from build123d import *

# Parameters (mm, degrees)
FILLET1_R               = 0.1
FILLET2_R               = 0.15
HEX_2_DEPTH             = 1.3
CUT_EXTRUDE1_DEPTH      = 14.569266765
CUT_EXTRUDE1_DEPTH_BACK = 14.569266765
SKETCH4_R               = 0.5


with BuildPart() as part:
    # BodySke → Base-Revolve (revolve)
    with BuildSketch(Plane.XY, mode=Mode.PRIVATE) as base_revolve_sk:
        Polygon((0, 0), (0, 2.75), (3, 2.75), (3, 1.5), (12.7195, 1.5), (13, 1.2195), (13, 0), align=None)
    revolve(base_revolve_sk.sketch.rotate(Axis((-31.75, 0, 0), (1, 0, 0)), 90), axis=Axis((-31.75, 0, 0), (1, 0, 0)))

    # Fillet1
    fillet1_edges = [part.edges().sort_by_distance(p)[0] for p in [
        (3, 0, -1.5),
    ]]
    fillet(fillet1_edges, radius=FILLET1_R)

    # Fillet2
    fillet2_edges = [part.edges().sort_by_distance(p)[0] for p in [
        (0, 0, -2.75),
    ]]
    fillet(fillet2_edges, radius=FILLET2_R)

    # Sketch2 → Hex-PreBroach (revolve, cut)
    with BuildSketch(Plane.XY, mode=Mode.PRIVATE) as hex_prebroach_sk:
        Polygon((0, 1.28), (1.3, 1.28), (2.039008345, 0), (0, 0), align=None)
    revolve(hex_prebroach_sk.sketch.rotate(Axis((0, 0, 0), (1, 0, 0)), 90), axis=Axis((0, 0, 0), (1, 0, 0)), mode=Mode.SUBTRACT)

    # Sketch3 → Hex 2 (cut)
    with BuildSketch(Plane(origin=(0, 0, 0), x_dir=(0, 0.500000000000001, 0.866025403784438), z_dir=(-1, 0, 0))):
        Polygon((0.739008345, 1.28), (-0.739008345, 1.28), (-1.478016689, 0), (-0.739008345, -1.28), (0.739008345, -1.28), (1.478016689, 0), align=None)
    extrude(amount=-HEX_2_DEPTH, mode=Mode.SUBTRACT)

    # Sketch4 → Cut-Extrude1 (cut, two sides: drawn at the far end of the back side and taken through both)
    with BuildSketch(Plane(origin=(0, 0, 0), x_dir=(1, 0, 0), z_dir=(0, 1, 0)).offset(-CUT_EXTRUDE1_DEPTH_BACK)):
        with Locations(Location((0.65, 0, 0), (0, 0, 180))):
            Circle(SKETCH4_R)
    extrude(amount=CUT_EXTRUDE1_DEPTH + CUT_EXTRUDE1_DEPTH_BACK, mode=Mode.SUBTRACT)


solid = part.part
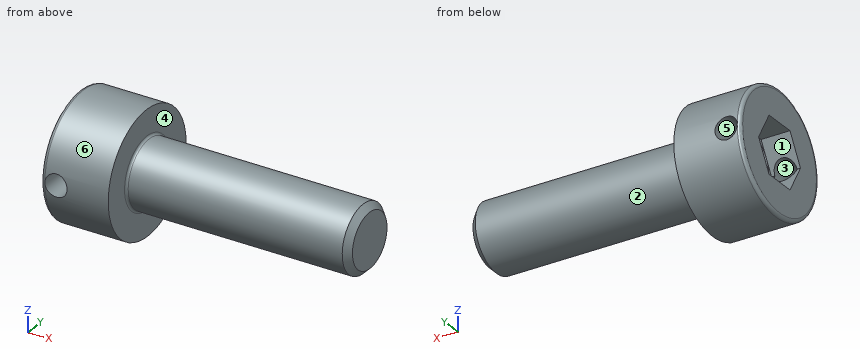
Can you work these out from the model? Positions are in its coordinate system, mm. Face numbers are marked on the shaded views. A direction names the side the tool comes from. Give positions to 0.01 mm unless a question says otherwise; leave off trailing zeros. Order: outer loops, then holes, each group sorted by start corner. A loop starts at its lowest first (then second) coordinate and runs counter-clockwise, first axis right, second up. Notation, with made-up numbers: (41, -21.75) - (88, -21.75) arc R23 ccw to (88, 11.25) - close; hole circle Ø8 at (-10.5, 73.25). An arc over 180 degrees is marked (long way). Write each question's results on one line, items separated by ' | '.
1) I'm going to push flat-ended pins straight in: pin 1 Ø2 at (x, y) = (6, 2) entering from -Z; pin 2 Ø0.5 at (y, z) = (-0.5, 1) entering from -X; pin 3 Ø3 at (x, y) = (11.5, -0.5) entering from -Z. Where does each tip first touch, or does it pass through?
Final values:
pin 1: stops at z = -1.12 | pin 2: stops at x = 1.3 | pin 3: stops at z = -1.5
2) On a 3-axis mill with a long thin cutter (end or side, diameter ignored), from which of +Z, -Z, +X, -X, +Y, -Y can I reach the whole of each face in a straight line? I mean the marked faces 1, 2 and 3. Say none if no direction works.
Final values:
face 1: -X | face 2: +X | face 3: +Y, -Y
3) Suppose I cut it at B-B, the plane x = 3.5. Write out the boundary of the cut face in (y, z).
Final values:
outline: circle Ø3 at (0, 0)
4) Suppose I cut it at A-A, the plane x = 0.65. Write out the boundary of the cut face in (y, z), then the cut area to 3 significant figures.
Final values:
outline: (-2.7, -0.5) arc R2.75 ccw to (2.7, -0.5) - (1.19, -0.5) - (0.74, -1.28) - (-0.74, -1.28) - (-1.19, -0.5) - close; (-2.7, 0.5) - (-1.19, 0.5) - (-0.74, 1.28) - (0.74, 1.28) - (1.19, 0.5) - (2.7, 0.5) arc R2.75 ccw to start | area: 15.3 mm^2
5) If we mould it in two halves opening along Z, with no side actions, what happens to the marked faces 4, 5 and 6? For each: pulls with the +Z half, pulls with the -Z half, needs draft (parallel to the pull), parting line crosses it, or undercut.
Final values:
face 4: needs draft | face 5: undercut | face 6: parting line crosses it
6) Please list where these lines run through material, in increasing order: line 1 along Z through (x, y) = (0.65, -2.3); line 2 along Z through (x, y) = (1, -2.3); line 3 along Y through (x, z) = (8.25, 1.3). Write a range as [from, to].
Final values:
line 1: z = [-1.51, -0.5], [0.5, 1.51] | line 2: z = [-1.51, -0.36], [0.36, 1.51] | line 3: y = [-0.75, 0.75]
